Design review of the part built by this model. Coordinates are the model's own, in mm. Face numbers are marked on the shaded views. A direction names the side the tool comes from. Coordinates: 2 decimals unless noted, no trailing zeros. Order: outer loops, then holes, each group sorted by start corner. A loop starts at its lowest first (then second) coordinate and runs counter-clockwise, first axis right, second up. Notation, with made-up numbers: (42.5, 56.5) -> (80.5, 56.5) arc R28 ccw to (80.5, 79.5) -> close; hole circle Ø8 at (62, -3.75). An arc over 180 degrees is marked (long way). Write item = value, one per line.
```python
from build123d import *

# Parameters (mm, degrees)
SKETCH1_R               = 30.1
SKETCH1_R_2             = 1.2
SKETCH1_R_3             = 6.75
BOSS_EXTRUDE1_DEPTH     = 2.5
SKETCH2_R               = 10.75
SKETCH2_R_2             = 6.75
BOSS_EXTRUDE2_DEPTH     = 15
CUT_EXTRUDE1_DEPTH      = 47.024667299
CUT_EXTRUDE1_DEPTH_BACK = 47.024667299
SKETCH3_R               = 1.6


with BuildPart() as part:
    # Sketch1 → Boss-Extrude1 (new body)
    with BuildSketch(Plane(origin=(0, 0, 0), x_dir=(1, 0, 0), z_dir=(0, 1, 0))):
        with Locations(Location((0, 0, 0), (0, 0, 270))):
            Circle(SKETCH1_R)
        with Locations(Location((-26, 0, 0), (0, 0, 270))):
            Circle(SKETCH1_R_2, mode=Mode.SUBTRACT)
        with Locations(Location((-8.034441854, 24.727469424, 0), (0, 0, 270))):
            Circle(SKETCH1_R_2, mode=Mode.SUBTRACT)
        with Locations(Location((21.034441854, 15.28241656, 0), (0, 0, 270))):
            Circle(SKETCH1_R_2, mode=Mode.SUBTRACT)
        with Locations(Location((21.034441854, -15.28241656, 0), (0, 0, 270))):
            Circle(SKETCH1_R_2, mode=Mode.SUBTRACT)
        with Locations(Location((-8.034441854, -24.727469424, 0), (0, 0, 270))):
            Circle(SKETCH1_R_2, mode=Mode.SUBTRACT)
        with Locations(Location((0, 0, 0), (0, 0, 270))):
            Circle(SKETCH1_R_3, mode=Mode.SUBTRACT)
    extrude(amount=BOSS_EXTRUDE1_DEPTH)

    # Sketch2 → Boss-Extrude2 (add)
    with BuildSketch(Plane(origin=(0, 2.5, 0), x_dir=(1, 0, 0), z_dir=(0, 1, 0))):
        with Locations(Location((0, 0, 0), (0, 0, 270))):
            Circle(SKETCH2_R)
        with Locations(Location((0, 0, 0), (0, 0, 270))):
            Circle(SKETCH2_R_2, mode=Mode.SUBTRACT)
    extrude(amount=BOSS_EXTRUDE2_DEPTH)

    # Sketch3 → Cut-Extrude1 (cut, two sides: drawn at the far end of the back side and taken through both)
    with BuildSketch(Plane.XY.offset(-CUT_EXTRUDE1_DEPTH_BACK)):
        with Locations((0, 12.5)):
            Circle(SKETCH3_R)
    extrude(amount=CUT_EXTRUDE1_DEPTH + CUT_EXTRUDE1_DEPTH_BACK, mode=Mode.SUBTRACT)


solid = part.part
```
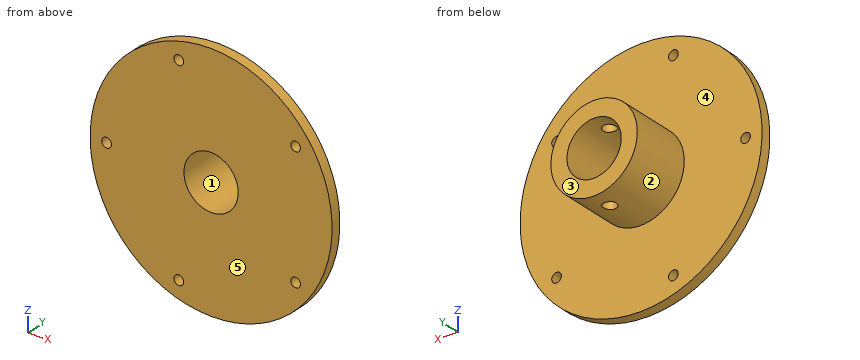
(1) We need section B-B (x = 0). Write out the cut boundary in (y, z), and give its area (3 significant figures).
Report:
outline = (0, -30.1) -> (2.5, -30.1) -> (2.5, -10.75) -> (10.9, -10.75) -> (10.9, -6.75) -> (0, -6.75) -> close; (0, 6.75) -> (10.9, 6.75) -> (10.9, 10.75) -> (2.5, 10.75) -> (2.5, 30.1) -> (0, 30.1) -> close; (14.1, -10.75) -> (17.5, -10.75) -> (17.5, -6.75) -> (14.1, -6.75) -> close; (14.1, 6.75) -> (17.5, 6.75) -> (17.5, 10.75) -> (14.1, 10.75) -> close
area = 211 mm²
(2) For the marked faces 4 and 5, list the 3-axis set-ups (+Z, -Z, +X, -X, +Y, -Y) from which the entire face can be reached by the end or side of a thin tool; tool diameter is ignored.
Report:
face_4 = +Y
face_5 = +Z, -Z, +X, -X, -Y
(3) The part is to be moulded in two halves that separate along Z. For the marked faces 1, 2 and 3, say which applies: released by +Z, released by -Z, zero draft, split by the parting line, or undercut.
Report:
face_1 = undercut
face_2 = split by the parting line
face_3 = zero draft
(4) For L1, parallel to X at y = 14, z = 0; L2, parallel to Y at x = 14, z = 10, list the stretches that pass through material, from the lowest coordinate up.
Report:
L1 = -10.75 to -6.75, 6.75 to 10.75
L2 = 0 to 2.5
(5) Insertion check: pin 1 (6 mm diameter, centred on y = 2.5, z = 11, fed in from +X); pin 2 (2 mm diameter, centred on x = -19, z = -19.5, fed in from +Y); pin 3 (3.5 mm diameter, centred on x = 0, y = 12.5, fed in from -Z); pin 4 (21.5 mm diameter, centred on x = 0, z = 0, fed in from -Y). Each pin has a flat end and moves straight along its axis. Give the tip position at first contact, or say it passes through.
Report:
pin_1 = 29.02
pin_2 = 2.5
pin_3 = -10.75
pin_4 = 0
(6) We need section D-D (y = 12.5). Write out the cut boundary in (x, z), and give its area (3 significant figures).
Report:
outline = (-1.6, -10.63) -> (-1.6, -6.56) arc R6.75 cw to (-1.6, 6.56) -> (-1.6, 10.63) arc R10.75 ccw to start; (1.6, -10.63) arc R10.75 ccw to (1.6, 10.63) -> (1.6, 6.56) arc R6.75 cw to (1.6, -6.56) -> close
area = 194 mm²
(7) We need section A-A (z = 0). Write out the cut boundary in (x, y), and give its area (3 significant figures).
Report:
outline = (-30.1, 0) -> (-27.2, 0) -> (-27.2, 2.5) -> (-30.1, 2.5) -> close; (-24.8, 0) -> (-6.75, 0) -> (-6.75, 17.5) -> (-10.75, 17.5) -> (-10.75, 2.5) -> (-24.8, 2.5) -> close; (6.75, 0) -> (30.1, 0) -> (30.1, 2.5) -> (10.75, 2.5) -> (10.75, 17.5) -> (6.75, 17.5) -> close
area = 231 mm²
(8) We need section C-C (x = -26). Write out the cut boundary in (y, z).
Report:
outline = (0, -15.17) -> (2.5, -15.17) -> (2.5, -1.2) -> (0, -1.2) -> close; (0, 1.2) -> (2.5, 1.2) -> (2.5, 15.17) -> (0, 15.17) -> close
